Input: part model. Units: mm. Frame: model coordinates. A direction names the side the tool comes from. Coordinates: 2 decimals unless noted, no trailing zeros. Order: outer loops, then holes, each group sorted by start corner. A loop starts at its lowest first (then second) coordinate and runs counter-clockwise, first axis right, second up. Notation, with made-up numbers: (-16.75, 54.25) -> (3.25, 54.25) arc R17 cw to (3.25, 82.25) -> close; hole circle Ø1 at (66.5, -27). An arc over 180 degrees is marked (long way). Answer as CSV lines item,"result".
from build123d import *

# Parameters (mm, degrees)
F2_DEPTH = 25


with BuildPart() as f2:
    # F0 (on Top) → F2 (new body)
    with BuildSketch(Plane.XY):
        with BuildLine():
            Line((-4.6122563072, 15), (-10, 15))
            ThreePointArc((-10, 15), (-17.0710678119, 12.0710678119), (-20, 5))
            Line((-20, 5), (-20, -5))
            ThreePointArc((-20, -5), (-17.0710678119, -12.0710678119), (-10, -15))
            Line((-10, -15), (10, -15))
            ThreePointArc((10, -15), (17.0710678119, -12.0710678119), (20, -5))
            Line((20, -5), (20, 5))
            ThreePointArc((20, 5), (17.0710678119, 12.0710678119), (10, 15))
            Line((10, 15), (4.6122563072, 15))
            add(Edge.make_bspline(
                [(4.6122563072, 15), (6.8289469928, 8.9060682803), (10.5117220245, 7.2656945751), (12.4788450791, -7.5751167321), (3.7502092309, -7.1033691056), (0, -7.3496685363)],
                knots=[0, 0, 0, 0, 0.3461122042, 0.6708599201, 1, 1, 1, 1], degree=3))
            add(Edge.make_bspline(
                [(-4.6122563072, 15), (-6.8289469928, 8.9060682803), (-10.5117220245, 7.2656945751), (-12.4788450791, -7.5751167321), (-3.7502092309, -7.1033691056), (0, -7.3496685363)],
                knots=[0, 0, 0, 0, 0.3461122042, 0.6708599201, 1, 1, 1, 1], degree=3))
        make_face()
    extrude(amount=F2_DEPTH)

    # F3: sweep along a path in F1
    with BuildLine(Plane.YZ) as f3_path:
        Line((0, 0), (0, 30))
        Line((0, 30), (-20.5212085995, 86.3815572472))
        Line((-20.5212085995, 86.3815572472), (-39.8048368901, 109.3628905407))
    # F0 (on Top) → F3 (sweep)
    with BuildSketch(Plane.XY):
        with BuildLine():
            Line((-4.6122563072, 15), (-10, 15))
            ThreePointArc((-10, 15), (-17.0710678119, 12.0710678119), (-20, 5))
            Line((-20, 5), (-20, -5))
            ThreePointArc((-20, -5), (-17.0710678119, -12.0710678119), (-10, -15))
            Line((-10, -15), (10, -15))
            ThreePointArc((10, -15), (17.0710678119, -12.0710678119), (20, -5))
            Line((20, -5), (20, 5))
            ThreePointArc((20, 5), (17.0710678119, 12.0710678119), (10, 15))
            Line((10, 15), (4.6122563072, 15))
            add(Edge.make_bspline(
                [(4.6122563072, 15), (6.8289469928, 8.9060682803), (10.5117220245, 7.2656945751), (12.4788450791, -7.5751167321), (3.7502092309, -7.1033691056), (0, -7.3496685363)],
                knots=[0, 0, 0, 0, 0.3461122042, 0.6708599201, 1, 1, 1, 1], degree=3))
            add(Edge.make_bspline(
                [(-4.6122563072, 15), (-6.8289469928, 8.9060682803), (-10.5117220245, 7.2656945751), (-12.4788450791, -7.5751167321), (-3.7502092309, -7.1033691056), (0, -7.3496685363)],
                knots=[0, 0, 0, 0, 0.3461122042, 0.6708599201, 1, 1, 1, 1], degree=3))
        make_face()
    sweep(path=f3_path.line, transition=Transition.RIGHT)


solid = f2.part
1. Cut plane A-A (x = -14). Return the cut outline in (y, z).
Findings:
outline,"(-50.66, 100.26) -> (-32.98, 79.19) -> (-14.17, 27.5) -> (-14.17, 0) -> (14.17, 0) -> (14.17, 32.5) -> (-8.06, 93.57) -> (-28.95, 118.47) -> close"
2. Cut plane B-B (x = 13). Return the cut outline in (y, z).
Findings:
outline,"(-50.94, 100.02) -> (-33.31, 79) -> (-14.54, 27.44) -> (-14.54, 0) -> (14.54, 0) -> (14.54, 32.56) -> (-7.74, 93.76) -> (-28.67, 118.71) -> close"
3. Reachability of faces 1 (the face through (-17.15, -11.99, 14.36)), 2 (the face through (0, -15, 13)), 3 (the face through (-7.27, -17.97, 106.68)), 4 (the face through (16.99, -12.15, 14.36)) from +Z, -Z, +X, -X, +Y, -Y: full face, straight path, thin tool, end or side. Return the list, or none.
Findings:
face 1,"-Z, -X, -Y"
face 2,"-Z, +X, -X, -Y"
face 3,"+Z, +X, -X, +Y"
face 4,"-Z, +X, -Y"
4. Ray query, line 1 along X through (y, z) = (-1, 30); line 2 along Y through (x, z) = (-8, 58); line 3 along X through (y, z) = (-4, 72.5). Return the intervals inside material, ascending.
Findings:
line 1,"x = -20 to -11.15, 11.15 to 20"
line 2,"y = -26.15 to -17, -1.29 to 5.77"
line 3,"x = -18.16 to -6.49, 6.49 to 18.16"
5. Contact query for flat-ended pins moving along their axis: pin 1 (8 mm diameter, centred on x = -6, y = 5, fed in from -Z); pin 2 (12 mm diameter, centred on x = 6.5, y = -6.5, fed in from +Z); pin 3 (10 mm diameter, centred on x = 1.5, z = 19.5, fed in from -Y); pin 4 (10 mm diameter, centred on x = -6, z = 41, fed in from +Y). Output: stop coordinate, or through.
Findings:
pin 1,"stops at z = 0"
pin 2,"stops at z = 100.16"
pin 3,"stops at y = -15"
pin 4,"stops at y = 13.78"
